The model under review builds one solid part; all positions refer to its coordinate system, in mm. A direction names the side the tool comes from. Round coordinates to 2 decimals unless told otherwise and drop trailing zeros. Order: outer loops, then holes, each group sorted by start corner. A loop starts at its lowest first (then second) coordinate and runs counter-clockwise, first axis right, second up.
1) Consider section C-C (z = 1.1). Give the boundary of the cut face in (x, y), then the cut area to 3 significant figures.
2) Consider section D-D (x = -12.5). Give the boundary of the cut face in (y, z).
3) Mouldability with a two-part tool opening along Y and no side actions: class faces 1 (the face through (0, 1, 2)), 2 (the face through (-1.63, -19.82, 3.04)), 3 (the face through (23.846, -7.509, 2.958)), 4 (the face through (0, 0, 6)) as pulls with the +Y half, pulls with the -Y half, needs draft (parallel to the pull), parting line crosses it, or undercut.
4) Consider section A-A (x = 0). Give the boundary of the cut face in (y, z).
5) To check wall thickness, follow L1, parallel to Y at x = 0, z = 4.75; L2, parallel to Y at x = 4.5, z = 1.95; L3, parallel to X at y = 2, z = 4.9. State the ranges of each line that lie inside material, in increasing order.
6) Machinability: for faces 5 (the face through (0, -1.5, 2)), 6 (the face through (5, -5, 0)), which of the approach directions +Z, -Z, +X, -X, +Y, -Y give a long, thin tool a straight path to every point of the face, cutting with its end or side? Answer none if there is none.
7) Clearance check with flat-ended pins moving along their axes: P1, Ø1.5, axis at y = -13, z = 0.5, coming from the -X side; P2, Ø0.7, axis at x = 0, z = 2.5, coming from the -Y side; P3, Ø2.5, axis at x = 0, y = -1, coming from the -Z side; P4, Ø2, axis at x = 18, z = 5, coming from the -Y side. State where each tip first meets the part, or that it passes through.
8) Consider section B-B (y = 0). Give the boundary of the cut face in (x, z).
Autodesk Inventor part; units mm, degrees
ref_plane "YZ Plane" through (0, 0, 0) normal (1, 0, 0) x (0, 1, 0)
ref_plane "XZ Plane" through (0, 0, 0) normal (0, 1, 0) x (-1, 0, 0)
ref_plane "XY Plane" through (0, 0, 0) normal (0, 0, 1) x (1, 0, 0)
sketch "Sketch1" plane through (0, 0, 0) normal (0, 0, 1) x (1, 0, 0)
  circle A0 centre (0, 0) radius 25
  arc A1 (-1.118, 1) -> (1.118, 1) centre (0, 0) ccw
  line L0 (0, 1) -> (1.118, 1)
  line L1 (1.118, 1) -> (0, 1)
  line L2 (0, 1) -> (-1.118, 1)
  dimension "d0" = 50
  dimension "d3" = 1
  dimension "d4" = 1.5
  dimension "d5" = 2.2361
  dimension "d6" = 1.118
extrude "Extrusion1" add sketch "Sketch1" along normal blind 4
sketch "Sketch2" plane through (0, 0, 4) normal (0, 0, 1) x (1, 0, 0)
  circle A0 centre (0, 0) radius 25
  circle A1 centre (0, 0) radius 25
extrude "Extrusion2" add sketch "Sketch2" along normal blind 2
sketch "Sketch3" plane through (0, 0, 0) normal (0, 0, -1) x (-1, 0, 0)
  point P0 (0, 0)
sketch "Sketch4" plane through (0, 0, 6) normal (0, 0, 1) x (1, 0, 0)
  circle A0 centre (12.5, 0) radius 7.5
  circle A1 centre (0, 12.5) radius 7.5
  circle A2 centre (-12.5, 0) radius 7.5
  circle A3 centre (0, -12.5) radius 7.5
  point P0 (0, 0)
  dimension "d14" = 15
  dimension "d15" = 12.5
  dimension "d18" = 360
extrude "Extrusion3" cut sketch "Sketch4" against normal through all
properties part number "wheel"
Answer below:
1. outline: circle Ø50 at (0, 0); hole circle Ø15 at (-12.5, 0); hole circle Ø15 at (0, -12.5); hole circle Ø15 at (0, 12.5); hole (-1.12, 1) arc R1.5 ccw (long way) to (1.12, 1) - close; hole circle Ø15 at (12.5, 0)
1. area: 1,250 mm2
2. outline: (-21.65, 0) - (-7.5, 0) - (-7.5, 6) - (-21.65, 6) - close; (7.5, 0) - (21.65, 0) - (21.65, 6) - (7.5, 6) - close
3. face 1: undercut
3. face 2: undercut
3. face 3: parting line crosses it
3. face 4: needs draft
4. outline: (-25, 0) - (-20, 0) - (-20, 6) - (-25, 6) - close; (-5, 0) - (-1.5, 0) - (-1.5, 4) - (1, 4) - (1, 0) - (5, 0) - (5, 6) - (-5, 6) - close; (20, 0) - (25, 0) - (25, 6) - (20, 6) - close
5. L1: y = -25 to -20, -5 to 5, 20 to 25
5. L2: y = -24.59 to -18.5, -6.5 to 6.5, 18.5 to 24.59
5. L3: x = -24.92 to -19.73, -5.27 to 5.27, 19.73 to 24.92
6. face 5: -Z
6. face 6: -Z, +X, -X, +Y, -Y
7. P1: stops at x = -21.79
7. P2: stops at y = -25
7. P3: stops at z = 0
7. P4: stops at y = -18.33
8. outline: (-25, 0) - (-20, 0) - (-20, 6) - (-25, 6) - close; (-5, 0) - (-1.5, 0) - (-1.5, 4) - (1.5, 4) - (1.5, 0) - (5, 0) - (5, 6) - (-5, 6) - close; (20, 0) - (25, 0) - (25, 6) - (20, 6) - close
